from build123d import *

# Parameters (mm, degrees)
SKETCH1_W           = 40.386
SKETCH1_H           = 18.796
BOSS_EXTRUDE1_DEPTH = 40.132
SKETCH2_W           = 7.239
SKETCH2_H           = 18.796
SKETCH2_R           = 2.5
BOSS_EXTRUDE2_DEPTH = 3.048
SKETCH3_R           = 3
BOSS_EXTRUDE3_DEPTH = 5.588


with BuildPart() as part:
    # Sketch1 → Boss-Extrude1 (new body)
    with BuildSketch(Plane(origin=(0, 0, 0), x_dir=(0, 0, -1), z_dir=(1, 0, 0))):
        with Locations((-20.193, -9.398)):
            Rectangle(SKETCH1_W, SKETCH1_H)
    extrude(amount=BOSS_EXTRUDE1_DEPTH)

    # Sketch2 → Boss-Extrude2 (add)
    with BuildSketch(Plane(origin=(26.924, 0, 0), x_dir=(0, 0, -1), z_dir=(1, 0, 0))):
        with Locations((-44.0055, -9.398)):
            Rectangle(SKETCH2_W, SKETCH2_H)
        with Locations((-44.323, -4.572)):
            Circle(SKETCH2_R, mode=Mode.SUBTRACT)
        with Locations((-44.323, -14.224)):
            Circle(SKETCH2_R, mode=Mode.SUBTRACT)
        with Locations((3.6195, -9.398)):
            Rectangle(SKETCH2_W, SKETCH2_H)
        with Locations((3.937, -4.572)):
            Circle(SKETCH2_R, mode=Mode.SUBTRACT)
        with Locations((3.937, -14.224)):
            Circle(SKETCH2_R, mode=Mode.SUBTRACT)
    extrude(amount=BOSS_EXTRUDE2_DEPTH)

    # Sketch3 → Boss-Extrude3 (add)
    with BuildSketch(Plane(origin=(40.132, 0, 0), x_dir=(0, 0, -1), z_dir=(1, 0, 0))):
        with Locations((-10.386, -9.398)):
            Circle(SKETCH3_R)
    extrude(amount=BOSS_EXTRUDE3_DEPTH)


solid = part.part
Read the model definition and answer for the solid it produces. Units are mm, in the model's axes. A direction names the side the tool comes from. Round coordinates to 2 decimals unless told otherwise and drop trailing zeros. Order: outer loops, then holes, each group sorted by start corner. A loop starts at its lowest first (then second) coordinate and runs counter-clockwise, first axis right, second up.
1) The part is cut by section A-A on y = -5.5. Write down the section's boundary in (x, z) (3 decimals), plus the area to 3 significant figures.
2) For faces 4 (the face through (26.924, -9, -4)), 5 (the face through (42.887, -9.266, 13.383)), 6 (the face through (13, -10, 40.386)), 7 (the face through (29.972, -9, 44)), 8 (the face through (35, -10, 0)), determine the directions among +Z, -Z, +X, -X, +Y, -Y from which every point of the face is accessible in a straight line to the end or side of a thin tool.
3) Straight lines are drawn through the part: L1, parallel to Z at x = 28.5, y = -14.5 (3 decimals); L2, parallel to Z at x = 30.5, y = -6; L3, parallel to X at y = -7, z = 17.5. For each, find the intervals that lie inside material, in ascending order.
4) The part is cut by section B-B on z = -4. Write down the section's boundary in (x, y).
5) The part is cut by section D-D on x = 10. Write down the section's boundary in (y, z), plus the area to 3 significant figures.
6) The part is cut by section C-C on y = -10.5. Write down the section's boundary in (x, z) (3 decimals).
7) The mould has two halves that part along Y. Classify faces 1 (the face through (26.924, -9, 44)), 2 (the face through (20, -18.796, 21)), 3 (the face through (28.427, -2.464, -5.281)): released by +Y, released by -Y, zero draft, split by the parting line, or undercut.
8) Flat-ended cylindrical pins translate along their axes: pin 1 (5.5 mm diameter, centred on x = 13, y = -5.5, fed in from -Z); pin 2 (9.5 mm diameter, centred on x = 20, y = -5.5, fed in from +Z); pin 3 (1 mm diameter, centred on y = -5, z = 30.5, fed in from +X). Find the tip coordinate at first contact, or state that the pin passes through.
Resolved:
1. outline: (0, 0) - (26.924, 0) - (26.924, -1.616) - (29.972, -1.616) - (29.972, 0) - (40.132, 0) - (40.132, 40.386) - (29.972, 40.386) - (29.972, 42.002) - (26.924, 42.002) - (26.924, 40.386) - (0, 40.386) - close; (26.924, -7.239) - (29.972, -7.239) - (29.972, -6.258) - (26.924, -6.258) - close; (26.924, 46.644) - (29.972, 46.644) - (29.972, 47.625) - (26.924, 47.625) - close
1. area: 1,640 mm2
2. face 4: -Z, -X, +Y, -Y
2. face 5: +X
2. face 6: +Z, -X, +Y, -Y
2. face 7: +Z, +X, +Y, -Y
2. face 8: -Z, +X, +Y, -Y
3. L1: z = -7.239 to -6.422, -1.452 to 41.838, 46.808 to 47.625
3. L2: z = 0 to 40.39
3. L3: x = 0 to 40.13
4. outline: (26.92, -18.8) - (29.97, -18.8) - (29.97, -16.72) - (26.92, -16.72) - close; (26.92, -11.72) - (29.97, -11.72) - (29.97, -7.07) - (26.92, -7.07) - close; (26.92, -2.07) - (29.97, -2.07) - (29.97, 0) - (26.92, 0) - close
5. outline: (-18.8, 0) - (0, 0) - (0, 40.39) - (-18.8, 40.39) - close
5. area: 759 mm2
6. outline: (0, 0) - (26.924, 0) - (26.924, -7.239) - (29.972, -7.239) - (29.972, 0) - (40.132, 0) - (40.132, 7.596) - (45.72, 7.596) - (45.72, 13.176) - (40.132, 13.176) - (40.132, 40.386) - (29.972, 40.386) - (29.972, 47.625) - (26.924, 47.625) - (26.924, 40.386) - (0, 40.386) - close
7. face 1: zero draft
7. face 2: released by -Y
7. face 3: undercut
8. pin 1: stops at z = 0
8. pin 2: stops at z = 40.39
8. pin 3: stops at x = 40.13
